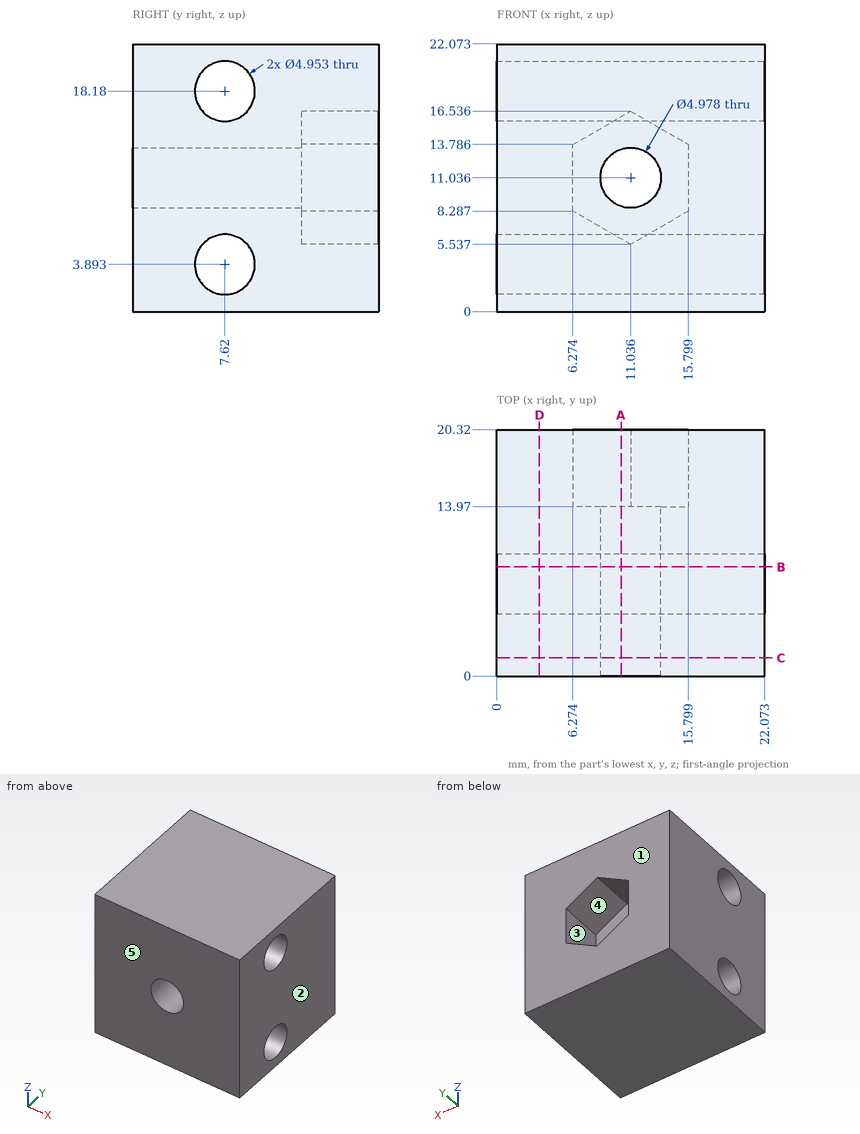
Could you check a few things on this drawing? It's one solid part, dimensions in mm from its lowest x, y, z. A direction names the side the tool comes from. Coordinates: 2 decimals unless noted, no trailing zeros. Order: outer loops, then holes, each group sorted by start corner. A loop starts at its lowest first (then second) coordinate and runs counter-clockwise, first axis right, second up. Notation, with made-up numbers: (-8.5, 35.25) - (37.5, 35.25) arc R22 ccw to (37.5, 58.25) - close; hole circle Ø7 at (-21.75, 7.25). An arc over 180 degrees is marked (long way). One line per question, with ' | ' between items.
(1) For the marked faces 4 and 5, which set-ups out of +Z, -Z, +X, -X, +Y, -Y let a thin tool reach every point of the face, with its end or its side?
Report:
face 4: +Y | face 5: +Z, -Z, +X, -X, -Y
(2) Suppose I cut it at B-B on y = 9. List the corners of the cut face in (x, z) for me (1 decimal), and give its area (3 significant figures).
Report:
outline: (0, 0) - (22.1, 0) - (22.1, 1.8) - (0, 1.8) - close; (0, 5.9) - (22.1, 5.9) - (22.1, 16.1) - (0, 16.1) - close; (0, 20.2) - (22.1, 20.2) - (22.1, 22.1) - (0, 22.1) - close; hole circle Ø5 at (11, 11) | area: 286 mm2
(3) If we mould it in two halves opening along X, with no side actions, what happens to the marked faces 1, 2 and 3? For each: pulls with the +X half, pulls with the -X half, needs draft (parallel to the pull), parting line crosses it, or undercut.
Report:
face 1: needs draft | face 2: pulls with the +X half | face 3: undercut
(4) If I drill on L1, parallel to Z at x = 5.25, y = 7.25 (1 decimal); L2, parallel to Y at x = 15.25, z = 3.75; L3, parallel to Z at x = 8.25, y = 18.75 (1 decimal), over which ranges is the centre line in solid material (lowest first)?
Report:
L1: z = 0 to 1.4, 6.3 to 15.7, 20.6 to 22.1 | L2: y = 0 to 5.15, 10.09 to 20.32 | L3: z = 0 to 7.1, 14.9 to 22.1
(5) Suppose I cut it at D-D on x = 3.5. List the corners of the cut face in (y, z) for me.
Report:
outline: (0, 0) - (20.32, 0) - (20.32, 22.07) - (0, 22.07) - close; hole circle Ø4.95 at (7.62, 3.89); hole circle Ø4.95 at (7.62, 18.18)
(6) Will this pin go through, and if not, where does the flat tip stop? pin 1 (5 mm diameter, centred on x = 10.5, z = 12, fed in from +Y).
Report:
pin 1: stops at y = 13.97
(7) Suppose I cut it at A-A on x = 10.25. List the corners of the cut face in (y, z) for me (1 decimal), and give its area (3 significant figures).
Report:
outline: (0, 0) - (20.3, 0) - (20.3, 6) - (14, 6) - (14, 8.7) - (0, 8.7) - close; (0, 13.4) - (14, 13.4) - (14, 16.1) - (20.3, 16.1) - (20.3, 22.1) - (0, 22.1) - close; hole circle Ø5 at (7.6, 3.9); hole circle Ø5 at (7.6, 18.2) | area: 280 mm2
(8) Suppose I cut it at C-C on y = 1.5. List the corners of the cut face in (x, z) for me (1 decimal), and give its area (3 significant figures).
Report:
outline: (0, 0) - (22.1, 0) - (22.1, 22.1) - (0, 22.1) - close; hole circle Ø5 at (11, 11) | area: 468 mm2
